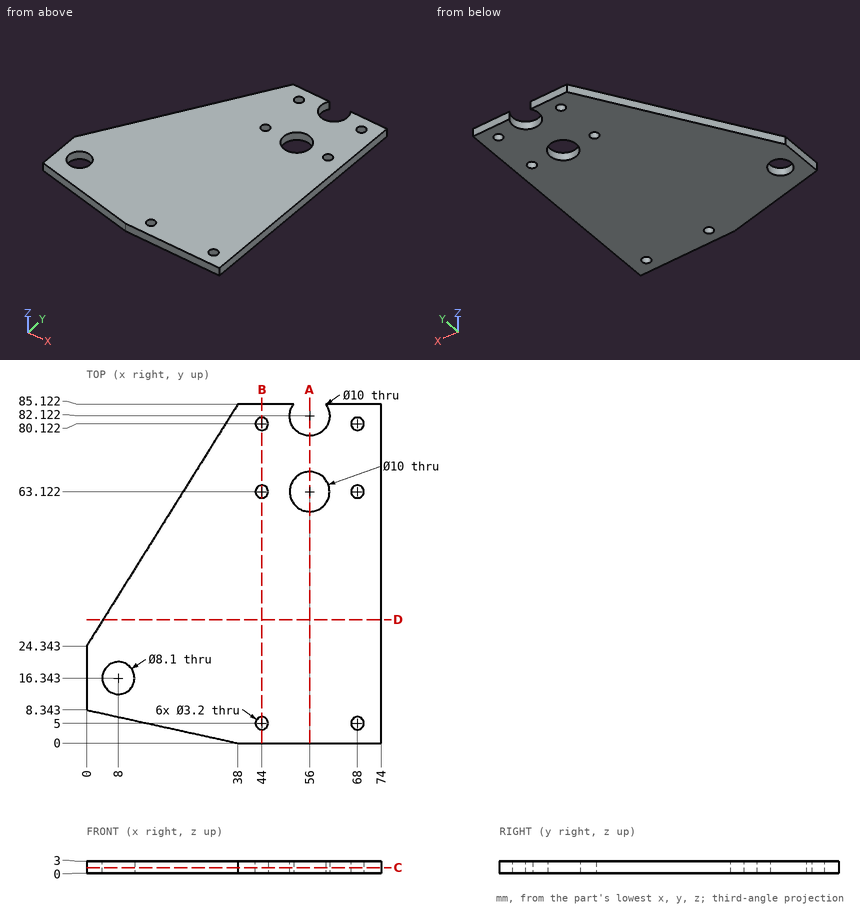
Print and shaded views of the part. All mm, measured from the part's lowest x, y and z. Coordinates: 2 decimals unless noted, no trailing zeros. Order: outer loops, then holes, each group sorted by start corner. A loop starts at its lowest first (then second) coordinate and runs counter-clockwise, first axis right, second up. Notation, with made-up numbers: (-30, 22) -> (19, 22) arc R10 cw to (19, 39) -> close; hole circle Ø9 at (7, -9). An arc over 180 degrees is marked (long way). Use one line per item in the form item = value. Start each with the question number.
1) Drop flat-ended pins along their axis: pin 1 (2.5 mm diameter, centred on x = 68, y = 80.12, fed in from +Z); pin 2 (1.5 mm diameter, centred on y = 50, z = 2.5, fed in from -X). Give the stop position or say it passes through.
2) Band-saw the part on A-A on x = 56. Give the cut face in (y, z), then the cut area to 3 significant figures.
3) Drill centre lines: L1, parallel to Y at x = 44, z = 0.55; L2, parallel to Y at x = 11.5, z = 0.3 (1 decimal); L3, parallel to X at y = 53.5, z = 0.4. Where is each one in solid material? Low to high. Write a range as [from, to].
4) Band-saw the part on B-B on x = 44. Give the cut face in (y, z).
5) Band-saw the part on C-C on z = 1.4. State how many separate pieces and enclosed holes the cut face has, then the cut area to 3 significant figures.
6) Band-saw the part on D-D on y = 31. Give the cut face in (x, z).
Entries:
q1.pin_1 = through
q1.pin_2 = 15.57
q2.outline = (0, 0) -> (58.12, 0) -> (58.12, 3) -> (0, 3) -> close; (68.12, 0) -> (77.12, 0) -> (77.12, 3) -> (68.12, 3) -> close
q2.area = 201 mm2
q3.L1 = [0, 3.4], [6.6, 61.52], [64.72, 78.52], [81.72, 85.12]
q3.L2 = [5.8, 14.3], [18.4, 42.7]
q3.L3 = [18.23, 74]
q4.outline = (0, 0) -> (3.4, 0) -> (3.4, 3) -> (0, 3) -> close; (6.6, 0) -> (61.52, 0) -> (61.52, 3) -> (6.6, 3) -> close; (64.72, 0) -> (78.52, 0) -> (78.52, 3) -> (64.72, 3) -> close; (81.72, 0) -> (85.12, 0) -> (85.12, 3) -> (81.72, 3) -> close
q5.separate_pieces = 1
q5.enclosed_holes = 8
q5.area = 4,740 mm2
q6.outline = (4.16, 0) -> (74, 0) -> (74, 3) -> (4.16, 3) -> close
